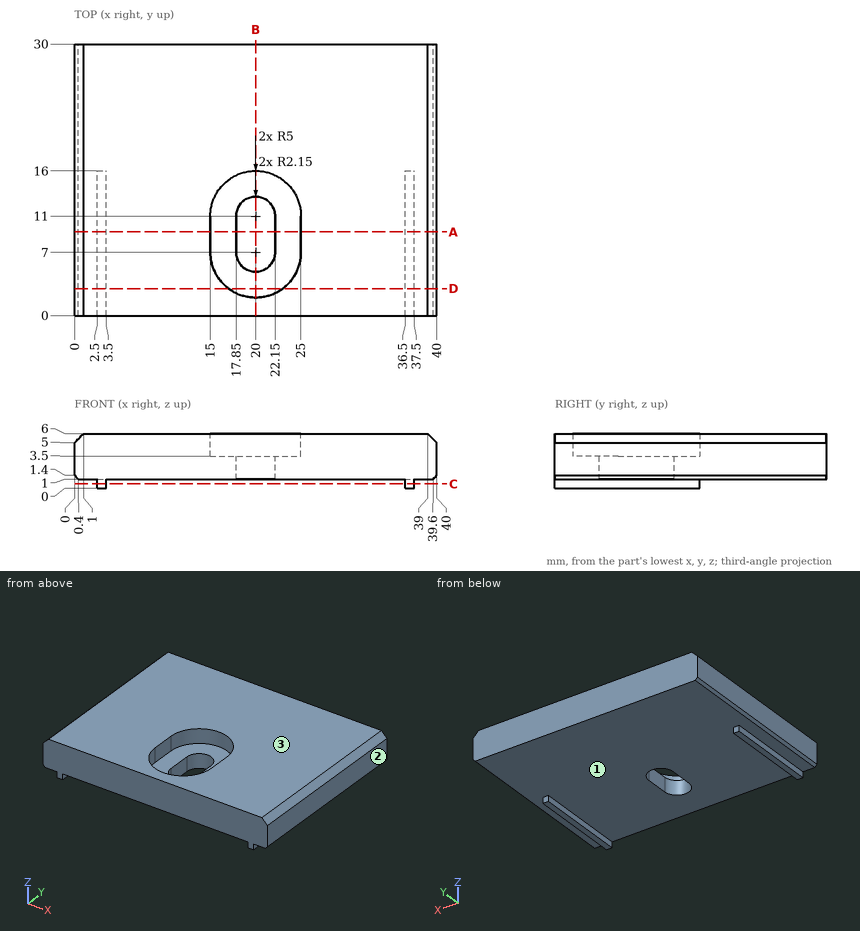
Geometry: see drawing. Coordinates: mm, zero at the bounding-box minimum. Give positions to 0.01 mm unless a question says otherwise; leave off trailing zeros. Order: outer loops, then holes, each group sorted by start corner. A loop starts at its lowest first (then second) coordinate and runs counter-clockwise, first axis right, second up.
1. Line query: probe 1 along X at (y, z) = (7.25, 2.2); probe 2 along X at (y, z) = (8.5, 4.2); probe 3 along Z at (x, y) = (23, 3.5). Output: solid intervals per line, ascending.
Computed:
probe 1: x = 0 to 17.85, 22.15 to 40
probe 2: x = 0 to 15, 25 to 40
probe 3: z = 1 to 3.5
2. Cut plane B-B (x = 20). Return loops of the section in (y, z), and give its area (4 significant figures).
Computed:
outline: (0, 1) - (4.85, 1) - (4.85, 3.5) - (2, 3.5) - (2, 6) - (0, 6) - close; (13.15, 1) - (30, 1) - (30, 6) - (16, 6) - (16, 3.5) - (13.15, 3.5) - close
area: 94.25 mm2
3. Cut plane A-A (y = 9.25). Return loops of the section in (x, z).
Computed:
outline: (0, 1.4) - (0.4, 1) - (2.5, 1) - (2.5, 0) - (3.5, 0) - (3.5, 1) - (17.85, 1) - (17.85, 3.5) - (15, 3.5) - (15, 6) - (1, 6) - (0, 5) - close; (22.15, 1) - (36.5, 1) - (36.5, 0) - (37.5, 0) - (37.5, 1) - (39.6, 1) - (40, 1.4) - (40, 5) - (39, 6) - (25, 6) - (25, 3.5) - (22.15, 3.5) - close
4. Cut plane D-D (y = 3). Return loops of the section in (x, z), and give its area (3 significant figures).
Computed:
outline: (0, 1.4) - (0.4, 1) - (2.5, 1) - (2.5, 0) - (3.5, 0) - (3.5, 1) - (36.5, 1) - (36.5, 0) - (37.5, 0) - (37.5, 1) - (39.6, 1) - (40, 1.4) - (40, 5) - (39, 6) - (23, 6) - (23, 3.5) - (17, 3.5) - (17, 6) - (1, 6) - (0, 5) - close
area: 186 mm2
5. Cut plane C-C (z = 0.45). Return loops of the section in (x, y).
Computed:
outline: (2.5, 0) - (3.5, 0) - (3.5, 16) - (2.5, 16) - close; (36.5, 0) - (37.5, 0) - (37.5, 16) - (36.5, 16) - close
6. Pin query (flat end, axial travel): pin 1 Ø0.5 at (y, z) = (10, 0.5) entering from -X; pin 2 Ø0.5 at (y, z) = (7, 0.5) entering from +X; pin 3 Ø15 at (x, y) = (26, 10.5) entering from -Z. Return the tip coordinate at first contact, or that it passes through.
Computed:
pin 1: stops at x = 2.5
pin 2: stops at x = 37.5
pin 3: stops at z = 1
7. Draft query along X for the marked faces 1, 2 and 3. Return one class per face: released by +X, released by -X, zero draft, split by the parting line, or undercut.
Computed:
face 1: undercut
face 2: released by +X
face 3: zero draft
